Input: part model. Units: mm. Frame: model coordinates. A direction names the side the tool comes from. Coordinates: 2 decimals unless noted, no trailing zeros. Order: outer loops, then holes, each group sorted by start corner. A loop starts at its lowest first (then second) coordinate and runs counter-clockwise, first axis right, second up. Notation, with made-up numbers: (79.5, 1.5) -> (126.5, 1.5) arc R15 ccw to (126.5, 25.5) -> close; hole circle Ø5 at (-3, -19). An arc over 180 degrees is marked (long way). Use CSV: the item, a comma, the result in double quotes. Start each with the question number.
```python
from build123d import *

# Parameters (mm, degrees)
F0_R        = 25.4
F0_R_2      = 17.914362
F1_DEPTH    = 4.572
F1_FACE_R   = 25.4
F1_FACE_R_2 = 17.914362
F2_DEPTH    = 4.572
F0_W        = 8.337361
F0_H        = 25.668724
F3_DEPTH    = 3.048
F4_DEPTH    = 3.048
F5_DEPTH    = 1.9812
F6_DEPTH    = 1.9812
F7_R        = 1.27
F8_R        = 0.367926


with BuildPart() as f1:
    # F0 (on Front) → F1 (new body)
    with BuildSketch(Plane.XZ):
        Circle(F0_R)
        Circle(F0_R_2, mode=Mode.SUBTRACT)
    extrude(amount=F1_DEPTH)

    # F1_face (on face) → F2 (join)
    with BuildSketch(Plane(origin=(0, 0, 0), x_dir=(1, 0, 0), z_dir=(0, 1, 0))):
        Circle(F1_FACE_R)
        Circle(F1_FACE_R_2, mode=Mode.SUBTRACT)
    extrude(amount=F2_DEPTH)

    # F0 (on Front) → F3 (join)
    with BuildSketch(Plane.XZ):
        Circle(F0_R_2)
        with Locations((0.105467, 0)):
            Rectangle(F0_W, F0_H, mode=Mode.SUBTRACT)
    extrude(amount=F3_DEPTH)

    # F0 (on Front) → F4 (join)
    with BuildSketch(Plane.XZ):
        Circle(F0_R_2)
        with Locations((0.105467, 0)):
            Rectangle(F0_W, F0_H, mode=Mode.SUBTRACT)
    extrude(amount=-F4_DEPTH)

    # F0 (on Front) → F5 (join)
    with BuildSketch(Plane.XZ):
        with Locations((0.105467, 0)):
            Rectangle(F0_W, F0_H)
    extrude(amount=F5_DEPTH)

    # F0 (on Front) → F6 (join)
    with BuildSketch(Plane.XZ):
        with Locations((0.105467, 0)):
            Rectangle(F0_W, F0_H)
    extrude(amount=-F6_DEPTH)

    # F7
    f7_edges = [f1.edges().sort_by_distance(p)[0] for p in [
        (-17.914362, 4.572, 0),
        (-25.4, 4.572, 0),
        (-25.4, -4.572, 0),
        (-17.914362, -4.572, 0),
    ]]
    fillet(f7_edges, radius=F7_R)

    # F8
    f8_edges = [f1.edges().sort_by_distance(p)[0] for p in [
        (0.105468, 3.048, -12.834362),
        (4.274148, 3.048, 0),
        (0.105468, 3.048, 12.834362),
        (-4.063213, 3.048, 0),
        (-4.063213, -3.048, 0),
        (0.105468, -3.048, 12.834362),
        (4.274148, -3.048, 0),
        (0.105468, -3.048, -12.834362),
    ]]
    fillet(f8_edges, radius=F8_R)


solid = f1.part
```
1. Material intervals for line 1 along Z through (x, y) = (0, 3.15); line 2 along Y through (x, z) = (-5, -14.5), sorted ascending.
2. Pull-direction query (X, two-part tool) for faces 1 (the face through (-16, -4.572, -11)), 2 (the face through (8, -3.048, 0)), 3 (the face through (-5.506, -0.046, 24.796)), 4 (the face through (8, 3.048, 0)); classes: released by +X, released by -X, zero draft, split by the parting line, or undercut.
3. Section C-C on y = 1.25. Return loops of the section in (x, z).
4. Access query for faces 5 (the face through (0, 1.981, 0)), 6 (the face through (-16, 4.572, 11)), 7 (the face through (0, -1.981, 0)). Directions: +Z, -Z, +X, -X, +Y, -Y. A direction counts if a zero-diameter tool reaches every point of the face in a straight line with its end or side. Return the directions, or none.
5. Contact query for flat-ended pins moving along their axis: P1, Ø5, axis at y = 3.5, z = 6, coming from the -X side; P2, Ø1, axis at x = 3, z = -17.5, coming from the -Y side; P3, Ø0.8, axis at x = 0, y = -2.5, coming from the +Z side. Output: stop coordinate, or through.
Values follow:
1,line 1,"z = -25.4 to -17.91, 17.91 to 25.4"
1,line 2,"y = -3.05 to 3.05"
2,face 1,"zero draft"
2,face 2,"undercut"
2,face 3,"split by the parting line"
2,face 4,"undercut"
3,outline,"circle Ø50.8 at (0, 0)"
4,face 5,"+Y"
4,face 6,"+Z, -Z, +X, -X, +Y"
4,face 7,"-Y"
5,P1,"stops at x = -25.16"
5,P2,"stops at y = -4.17"
5,P3,"stops at z = 25.4"
